Verification items for the finished model (mm, model axes). Face numbers are marked on the shaded views. Coordinates: 2 decimals unless noted, no trailing zeros. Write each loop counter-clockwise with the first axis right and the second up, starting at its lowest first coordinate (ties: lowest second). Pieces come first, ordered by that corner, then holes. Notation, with made-up numbers: (21.5, 11) -> (57.5, 11) arc R17 ccw to (57.5, 29) -> close; hole circle Ø8 at (43.5, 4). An arc over 180 degrees is marked (long way). Answer in a Markdown table with one row per item.
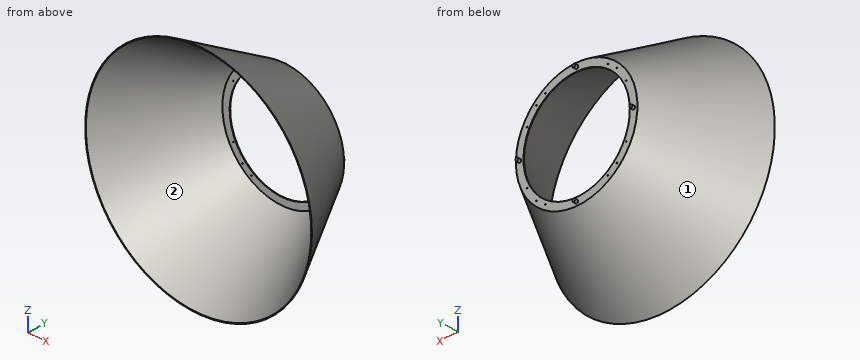
```python
from build123d import *

# Parameters (mm, degrees)
SKETCH2_R           = 200
BOSS_EXTRUDE1_DEPTH = 300
BOSS_EXTRUDE1_DRAFT = -30
SHELL1_T            = -2
CUT_EXTRUDE1_REACH  = 1631.392
SKETCH3_R           = 1.5
SKETCH3_R_2         = 175
SKETCH4_R           = 5.1
BOSS_EXTRUDE2_DEPTH = 10
CUT_EXTRUDE4_REACH  = 1631.392
SKETCH5_R           = 1.5


with BuildPart() as part:
    # Sketch2 → Boss-Extrude1 (with draft: the straight prism first)
    with BuildSketch(Plane.XZ.offset(-263.664131829)):
        with Locations((394.086664394, 1032.562454189)):
            Circle(SKETCH2_R)
    extrude(amount=BOSS_EXTRUDE1_DEPTH)
    # Boss-Extrude1: the draft: its side faces are tilted about the plane it starts from
    boss_extrude1_sides = [part.faces().sort_by_distance(p)[0] for p in [
        (194.086664394, 113.664131829, 1032.562454189),
    ]]
    draft(boss_extrude1_sides, Plane.XZ.offset(-263.664131829), BOSS_EXTRUDE1_DRAFT)

    # Shell1
    shell1_openings = [part.faces().sort_by_distance(p)[0] for p in [
        (394.086664394, -36.335868171, 1032.562454189),
    ]]
    offset(amount=SHELL1_T, openings=shell1_openings, kind=Kind.INTERSECTION)

    # Sketch3 → Cut-Extrude1 (cut, up to next)
    with BuildSketch(Plane(origin=(0, 263.664131829, 0), x_dir=(1, 0, 0), z_dir=(0, 1, 0)), mode=Mode.PRIVATE) as cut_extrude1_sk1:
        with Locations(Location((261.504142922, -1165.144975661, 0), (0, 0, 270))):
            Circle(SKETCH3_R)
    cut_extrude1_tool1 = extrude(cut_extrude1_sk1.sketch, amount=-CUT_EXTRUDE1_REACH, mode=Mode.PRIVATE) & part.part
    # Sketch3 → Cut-Extrude1 (cut, up to next)
    with BuildSketch(Plane(origin=(0, 263.664131829, 0), x_dir=(1, 0, 0), z_dir=(0, 1, 0)), mode=Mode.PRIVATE) as cut_extrude1_sk2:
        with Locations(Location((526.669185867, -1165.144975661, 0), (0, 0, 270))):
            Circle(SKETCH3_R)
    cut_extrude1_tool2 = extrude(cut_extrude1_sk2.sketch, amount=-CUT_EXTRUDE1_REACH, mode=Mode.PRIVATE) & part.part
    # Sketch3 → Cut-Extrude1 (cut, up to next)
    with BuildSketch(Plane(origin=(0, 263.664131829, 0), x_dir=(1, 0, 0), z_dir=(0, 1, 0)), mode=Mode.PRIVATE) as cut_extrude1_sk3:
        with Locations(Location((526.669185867, -899.979932716, 0), (0, 0, 270))):
            Circle(SKETCH3_R)
    cut_extrude1_tool3 = extrude(cut_extrude1_sk3.sketch, amount=-CUT_EXTRUDE1_REACH, mode=Mode.PRIVATE) & part.part
    # Sketch3 → Cut-Extrude1 (cut, up to next)
    with BuildSketch(Plane(origin=(0, 263.664131829, 0), x_dir=(1, 0, 0), z_dir=(0, 1, 0)), mode=Mode.PRIVATE) as cut_extrude1_sk4:
        with Locations(Location((261.504142922, -899.979932716, 0), (0, 0, 270))):
            Circle(SKETCH3_R)
    cut_extrude1_tool4 = extrude(cut_extrude1_sk4.sketch, amount=-CUT_EXTRUDE1_REACH, mode=Mode.PRIVATE) & part.part
    # Sketch3 → Cut-Extrude1 (cut, up to next)
    with BuildSketch(Plane(origin=(0, 263.664131829, 0), x_dir=(1, 0, 0), z_dir=(0, 1, 0)), mode=Mode.PRIVATE) as cut_extrude1_sk5:
        with Locations(Location((394.086664394, -1032.562454189, 0), (0, 0, 270))):
            Circle(SKETCH3_R_2)
    cut_extrude1_tool5 = extrude(cut_extrude1_sk5.sketch, amount=-CUT_EXTRUDE1_REACH, mode=Mode.PRIVATE) & part.part
    add(cut_extrude1_tool1.solids().sort_by_distance((261.504143, 263.664132, 1165.144976))[0], mode=Mode.SUBTRACT)
    add(cut_extrude1_tool2.solids().sort_by_distance((526.669186, 263.664132, 1165.144976))[0], mode=Mode.SUBTRACT)
    add(cut_extrude1_tool3.solids().sort_by_distance((526.669186, 263.664132, 899.979933))[0], mode=Mode.SUBTRACT)
    add(cut_extrude1_tool4.solids().sort_by_distance((261.504143, 263.664132, 899.979933))[0], mode=Mode.SUBTRACT)
    add(cut_extrude1_tool5.solids().sort_by_distance((394.086664, 263.664132, 1032.562454))[0], mode=Mode.SUBTRACT)

    # Sketch4 → Boss-Extrude2 (add)
    with BuildSketch(Plane(origin=(0, 263.664131829, 0), x_dir=(1, 0, 0), z_dir=(0, 1, 0))):
        with Locations(Location((206.586664394, -1032.562454189, 0), (0, 0, 90))):
            Circle(SKETCH4_R)
        with Locations(Location((394.086664394, -845.062454189, 0), (0, 0, 90))):
            Circle(SKETCH4_R)
        with Locations(Location((581.586664394, -1032.562454189, 0), (0, 0, 90))):
            Circle(SKETCH4_R)
        with Locations(Location((394.086664394, -1220.062454189, 0), (0, 0, 90))):
            Circle(SKETCH4_R)
    extrude(amount=BOSS_EXTRUDE2_DEPTH)

    # Sketch5 → Cut-Extrude4 (cut, up to next)
    with BuildSketch(Plane(origin=(0, 263.664131829, 0), x_dir=(1, 0, 0), z_dir=(0, 1, 0)), mode=Mode.PRIVATE) as cut_extrude4_sk1:
        with Locations(Location((231.086664394, -1117.562454189, 0), (0, 0, 270))):
            Circle(SKETCH5_R)
    cut_extrude4_tool1 = extrude(cut_extrude4_sk1.sketch, amount=-CUT_EXTRUDE4_REACH, mode=Mode.PRIVATE) & part.part
    # Sketch5 → Cut-Extrude4 (cut, up to next)
    with BuildSketch(Plane(origin=(0, 263.664131829, 0), x_dir=(1, 0, 0), z_dir=(0, 1, 0)), mode=Mode.PRIVATE) as cut_extrude4_sk2:
        with Locations(Location((557.086664394, -1117.562454189, 0), (0, 0, 270))):
            Circle(SKETCH5_R)
    cut_extrude4_tool2 = extrude(cut_extrude4_sk2.sketch, amount=-CUT_EXTRUDE4_REACH, mode=Mode.PRIVATE) & part.part
    # Sketch5 → Cut-Extrude4 (cut, up to next)
    with BuildSketch(Plane(origin=(0, 263.664131829, 0), x_dir=(1, 0, 0), z_dir=(0, 1, 0)), mode=Mode.PRIVATE) as cut_extrude4_sk3:
        with Locations(Location((497.086664394, -1187.562454189, 0), (0, 0, 270))):
            Circle(SKETCH5_R)
    cut_extrude4_tool3 = extrude(cut_extrude4_sk3.sketch, amount=-CUT_EXTRUDE4_REACH, mode=Mode.PRIVATE) & part.part
    # Sketch5 → Cut-Extrude4 (cut, up to next)
    with BuildSketch(Plane(origin=(0, 263.664131829, 0), x_dir=(1, 0, 0), z_dir=(0, 1, 0)), mode=Mode.PRIVATE) as cut_extrude4_sk4:
        with Locations(Location((557.086664394, -947.562454189, 0), (0, 0, 270))):
            Circle(SKETCH5_R)
    cut_extrude4_tool4 = extrude(cut_extrude4_sk4.sketch, amount=-CUT_EXTRUDE4_REACH, mode=Mode.PRIVATE) & part.part
    # Sketch5 → Cut-Extrude4 (cut, up to next)
    with BuildSketch(Plane(origin=(0, 263.664131829, 0), x_dir=(1, 0, 0), z_dir=(0, 1, 0)), mode=Mode.PRIVATE) as cut_extrude4_sk5:
        with Locations(Location((497.086664394, -877.562454189, 0), (0, 0, 270))):
            Circle(SKETCH5_R)
    cut_extrude4_tool5 = extrude(cut_extrude4_sk5.sketch, amount=-CUT_EXTRUDE4_REACH, mode=Mode.PRIVATE) & part.part
    # Sketch5 → Cut-Extrude4 (cut, up to next)
    with BuildSketch(Plane(origin=(0, 263.664131829, 0), x_dir=(1, 0, 0), z_dir=(0, 1, 0)), mode=Mode.PRIVATE) as cut_extrude4_sk6:
        with Locations(Location((291.086664394, -877.562454189, 0), (0, 0, 270))):
            Circle(SKETCH5_R)
    cut_extrude4_tool6 = extrude(cut_extrude4_sk6.sketch, amount=-CUT_EXTRUDE4_REACH, mode=Mode.PRIVATE) & part.part
    # Sketch5 → Cut-Extrude4 (cut, up to next)
    with BuildSketch(Plane(origin=(0, 263.664131829, 0), x_dir=(1, 0, 0), z_dir=(0, 1, 0)), mode=Mode.PRIVATE) as cut_extrude4_sk7:
        with Locations(Location((231.086664394, -947.562454189, 0), (0, 0, 270))):
            Circle(SKETCH5_R)
    cut_extrude4_tool7 = extrude(cut_extrude4_sk7.sketch, amount=-CUT_EXTRUDE4_REACH, mode=Mode.PRIVATE) & part.part
    # Sketch5 → Cut-Extrude4 (cut, up to next)
    with BuildSketch(Plane(origin=(0, 263.664131829, 0), x_dir=(1, 0, 0), z_dir=(0, 1, 0)), mode=Mode.PRIVATE) as cut_extrude4_sk8:
        with Locations(Location((291.086664394, -1187.562454189, 0), (0, 0, 270))):
            Circle(SKETCH5_R)
    cut_extrude4_tool8 = extrude(cut_extrude4_sk8.sketch, amount=-CUT_EXTRUDE4_REACH, mode=Mode.PRIVATE) & part.part
    add(cut_extrude4_tool1.solids().sort_by_distance((231.086664, 263.664132, 1117.562454))[0], mode=Mode.SUBTRACT)
    add(cut_extrude4_tool2.solids().sort_by_distance((557.086664, 263.664132, 1117.562454))[0], mode=Mode.SUBTRACT)
    add(cut_extrude4_tool3.solids().sort_by_distance((497.086664, 263.664132, 1187.562454))[0], mode=Mode.SUBTRACT)
    add(cut_extrude4_tool4.solids().sort_by_distance((557.086664, 263.664132, 947.562454))[0], mode=Mode.SUBTRACT)
    add(cut_extrude4_tool5.solids().sort_by_distance((497.086664, 263.664132, 877.562454))[0], mode=Mode.SUBTRACT)
    add(cut_extrude4_tool6.solids().sort_by_distance((291.086664, 263.664132, 877.562454))[0], mode=Mode.SUBTRACT)
    add(cut_extrude4_tool7.solids().sort_by_distance((231.086664, 263.664132, 947.562454))[0], mode=Mode.SUBTRACT)
    add(cut_extrude4_tool8.solids().sort_by_distance((291.086664, 263.664132, 1187.562454))[0], mode=Mode.SUBTRACT)


solid = part.part
```
1. Thickness scan on line 1 (Y direction, x = 584, z = 1067); line 2 (Z direction, x = 334.5, y = 134); line 3 (X direction, y = 182.5, z = 908). Record the ranges inside material, lowest first. Write a range as from..to.
Geometry says:
| item | result |
|---|---|
| line 1 | 261.66..263.66 |
| line 2 | 764.24..766.6, 1298.52..1300.89 |
| line 3 | 180.96..183.64, 604.54..607.22 |
2. Mould release check, pull along Z, two halves, no side actions. Record for the marked faces 1 and 2: released by +Z, released by -Z, zero draft, split by the parting line, or undercut.
Geometry says:
| item | result |
|---|---|
| face 1 | split by the parting line |
| face 2 | undercut |
3. Section check B-B, the plane y = 68.5. Record the boundary of the cut face in (x, z).
Geometry says:
| item | result |
|---|---|
| outline | circle Ø625.36 at (394.09, 1032.56); hole circle Ø620.74 at (394.09, 1032.56) |
4. Section check A-A, the plane y = 159.5. Record the boundary of the cut face in (x, z).
Geometry says:
| item | result |
|---|---|
| outline | circle Ø520.28 at (394.09, 1032.56); hole circle Ø515.66 at (394.09, 1032.56) |
5. Depth check by flat-ended pin: P1, Ø4, axis at x = 231.09, z = 1117.56, coming from the +Y side; P2, Ø12, axis at y = 195, z = 1145, coming from the -X side; P3, Ø5, axis at x = 291.09, z = 1187.56, coming from the -Y side. Enter the tip coordinate at first touch or a pass-through.
Geometry says:
| item | result |
|---|---|
| P1 | y = 263.66 |
| P2 | x = 177.48 |
| P3 | y = 261.66 |
